```python
from build123d import *

# Parameters (mm, degrees)
SKETCH1_W           = 20
SKETCH1_H           = 16
BOSS_EXTRUDE1_DEPTH = 13
SKETCH2_W           = 20
SKETCH2_H           = 8
CUT_EXTRUDE1_DEPTH  = 3.6
SKETCH3_R           = 1.8
CUT_EXTRUDE2_DEPTH  = 17
BOSS_EXTRUDE2_DEPTH = 2
BOSS_EXTRUDE3_DEPTH = 13
SKETCH7_W           = 20
SKETCH7_H           = 8
CUT_EXTRUDE3_DEPTH  = 4
FILLET1_R           = 0.5
SKETCH8_R           = 3.245
CUT_EXTRUDE4_DEPTH  = 14.0000001


with BuildPart() as part:
    # Sketch1 → Boss-Extrude1 (new body)
    with BuildSketch(Plane.XY):
        with Locations((10, 8)):
            Rectangle(SKETCH1_W, SKETCH1_H)
    extrude(amount=BOSS_EXTRUDE1_DEPTH)

    # Sketch2 → Cut-Extrude1 (cut)
    with BuildSketch(Plane.XZ):
        with Locations((10, 6.5)):
            Rectangle(SKETCH2_W, SKETCH2_H)
    extrude(amount=-CUT_EXTRUDE1_DEPTH, mode=Mode.SUBTRACT)

    # Sketch3 → Cut-Extrude2 (cut, through all)
    with BuildSketch(Plane(origin=(0, 16, 0), x_dir=(1, 0, 0), z_dir=(0, 1, 0))):
        with Locations((3.3, -6.5)):
            Circle(SKETCH3_R)
        with Locations((16.7, -6.5)):
            Circle(SKETCH3_R)
    extrude(amount=-CUT_EXTRUDE2_DEPTH, mode=Mode.SUBTRACT)

    # Sketch4 → Boss-Extrude2 (add)
    with BuildSketch(Plane.XZ.offset(-3.6)):
        Polygon((7.601093671, 8.983237589), (4.973984112, 10.5), (1.626015888, 10.5), (0, 9.561219289), (0, 3.438780711), (1.626015888, 2.5), (4.973984112, 2.5), (7.601093671, 4.016762411), align=None)
        Polygon((0.498906329, 8.117212185), (3.3, 9.73442437), (6.101093671, 8.117212185), (6.101093671, 4.882787815), (3.3, 3.26557563), (0.498906329, 4.882787815), align=None, mode=Mode.SUBTRACT)
        Polygon((18.373984112, 10.5), (15.026015888, 10.5), (12.398906329, 8.983237589), (12.398906329, 4.016762411), (15.026015888, 2.5), (18.373984112, 2.5), (20, 3.438780711), (20, 9.561219289), align=None)
        Polygon((13.898906329, 8.117212185), (16.7, 9.73442437), (19.501093671, 8.117212185), (19.501093671, 4.882787815), (16.7, 3.26557563), (13.898906329, 4.882787815), align=None, mode=Mode.SUBTRACT)
    extrude(amount=BOSS_EXTRUDE2_DEPTH)

    # Sketch6 → Boss-Extrude3 (add)
    with BuildSketch(Plane.XY.offset(13)):
        Polygon((0.1, 0), (0.1, -2.4), (2.843031442, -2.4), (1.743600076, -0.042261826), (1.723893063, 0), align=None)
        Polygon((12.843031442, -2.4), (11.743600076, -0.042261826), (11.723893063, 0), (8.276106937, 0), (8.256399924, -0.042261826), (7.156968558, -2.4), align=None)
        Polygon((19.9, -2.4), (19.9, 0), (18.276106937, 0), (18.256399924, -0.042261826), (17.156968558, -2.4), align=None)
    extrude(amount=-BOSS_EXTRUDE3_DEPTH)

    # Sketch7 → Cut-Extrude3 (cut)
    with BuildSketch(Plane.XZ.offset(2.4)):
        with Locations((10, 6.5)):
            Rectangle(SKETCH7_W, SKETCH7_H)
    extrude(amount=-CUT_EXTRUDE3_DEPTH, mode=Mode.SUBTRACT)

    # Fillet1
    fillet1_edges = [part.edges().sort_by_distance(p)[0] for p in [
        (1.723893063, 0, 1.25),
        (1.723893063, 0, 11.75),
        (8.276106937, 0, 1.25),
        (11.723893063, 0, 1.25),
        (11.723893063, 0, 11.75),
        (8.276106937, 0, 11.75),
        (18.276106937, 0, 1.25),
        (18.276106937, 0, 11.75),
    ]]
    fillet(fillet1_edges, radius=FILLET1_R)

    # Sketch8 → Cut-Extrude4 (cut, through all)
    with BuildSketch(Plane.XY.offset(13)):
        with Locations((10, 8)):
            Circle(SKETCH8_R)
    extrude(amount=-CUT_EXTRUDE4_DEPTH, mode=Mode.SUBTRACT)


solid = part.part
```
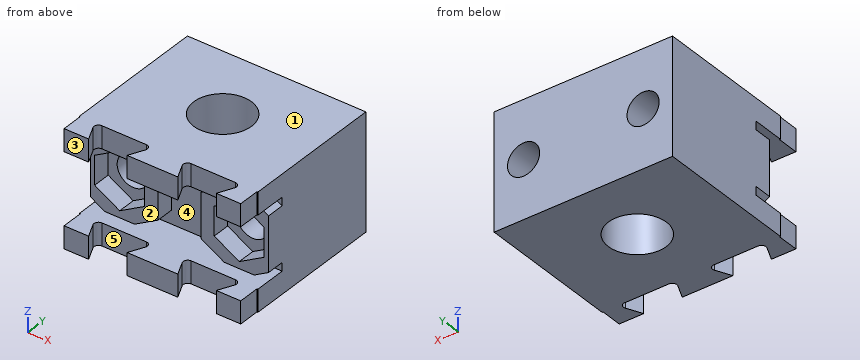
Input: part model. Units: mm. Frame: model coordinates. Face numbers are marked on the shaded views. A direction names the side the tool comes from. Give positions to 0.01 mm unless a question says otherwise; leave off trailing zeros. Order: outer loops, then holes, each group sorted by start corner. A loop starts at its lowest first (then second) coordinate and runs counter-clockwise, first axis right, second up. Notation, with made-up numbers: M -9,28.25 L 2,28.25 A17 cw 2,53.25 Z; hole C -2,-0.5 d6. An arc over 180 degrees is marked long. Return JSON: item names as keys, results as strings.
1) Mould query, pull axis Z, two halves, no side actions, for the marked faces 1, 2 and 3. Classes: released by +Z, released by -Z, zero draft, split by the parting line, or undercut.
Taken from the geometry:
{"face 1": "released by +Z", "face 2": "undercut", "face 3": "zero draft"}
2) Section query C-C on x = 10. Output: boundary loops of the cut face in (y, z) (3 decimals).
Taken from the geometry:
{"outline": "M -2.4,0 L 4.755,0 L 4.755,13 L -2.4,13 L -2.4,10.5 L 3.6,10.5 L 3.6,2.5 L -2.4,2.5 Z; M 11.245,0 L 16,0 L 16,13 L 11.245,13 Z"}
3) Section query A-A on z = 6.5. Output: boundary loops of the cut face in (x, y) (3 decimals).
Taken from the geometry:
{"outline": "M 0,1.6 L 0.499,1.6 L 0.499,3.6 L 1.5,3.6 L 1.5,16 L 0,16 Z; M 5.1,3.6 L 6.101,3.6 L 6.101,1.6 L 7.601,1.6 L 7.601,3.6 L 12.399,3.6 L 12.399,1.6 L 13.899,1.6 L 13.899,3.6 L 14.9,3.6 L 14.9,16 L 5.1,16 Z; M 18.5,3.6 L 19.501,3.6 L 19.501,1.6 L 20,1.6 L 20,16 L 18.5,16 Z; hole C 10,8 d6.49"}
4) Access query for the marked faces 4 and 5. Directions: +Z, -Z, +X, -X, +Y, -Y. A direction counts if a zero-diameter tool reaches every point of the face in a straight line with its end or side. Return the directions, or none.
Taken from the geometry:
{"face 4": "-Y", "face 5": "+Z, -Z"}
5) Contact query for flat-ended pins moving along their axis: pin 1 (4.5 mm diameter, centred on x = 17.5, z = 7.5, fed in from -Y); pin 2 (1.3 mm diameter, centred on x = 4, z = 1, fed in from -Y); pin 3 (1.9 mm diameter, centred on y = -1, z = 1.5, fed in from -X). Output: stop coordinate, or through.
Taken from the geometry:
{"pin 1": "stops at y = 1.6", "pin 2": "stops at y = 0", "pin 3": "stops at x = 0.1"}
6) Section query D-D on y = 4.5. Output: boundary loops of the cut face in (x, z).
Taken from the geometry:
{"outline": "M 0,0 L 20,0 L 20,13 L 0,13 Z; hole C 3.3,6.5 d3.6; hole C 16.7,6.5 d3.6"}
7) Section query B-B on y = 8. Output: boundary loops of the cut face in (x, z) (3 decimals), and give its area (3 significant figures).
Taken from the geometry:
{"outline": "M 0,0 L 6.755,0 L 6.755,13 L 0,13 Z; M 13.245,0 L 20,0 L 20,13 L 13.245,13 Z; hole C 3.3,6.5 d3.6; hole C 16.7,6.5 d3.6", "area": "155 mm2"}
8) Line query: L1, parallel to X at y = 11.5, z = 6.5; L2, parallel to Y at x = 10, z = 9.25 (3 decimals); L3, parallel to Z at x = 10.75, y = 2.75. Output: solid intervals per line, ascending. Write a range as [from, to].
Taken from the geometry:
{"L1": "x = [0, 1.5], [5.1, 14.9], [18.5, 20]", "L2": "y = [3.6, 4.755], [11.245, 16]", "L3": "z = [0, 2.5], [10.5, 13]"}
